from build123d import *

# Parameters (mm, degrees)
BOSS_EXTRUDE1_DEPTH = 11.1125
SKETCH3_W           = 6.35
SKETCH3_H           = 6.35
CUT_EXTRUDE1_DEPTH  = 6.35
SKETCH2_R           = 1.5875
CUT_EXTRUDE2_DEPTH  = 3.175
CUT_EXTRUDE3_REACH  = 19.451
SKETCH4_R           = 1.7859375


with BuildPart() as part:
    # Sketch1 → Boss-Extrude1 (new body)
    with BuildSketch(Plane.XY):
        Polygon((0, 0), (0, 7.62), (12.7, 7.62), (12.7, 4.445), (6.35, 4.445), (6.35, 0), align=None)
    extrude(amount=BOSS_EXTRUDE1_DEPTH)

    # Mirror1: part across plane


with BuildPart() as part_1:
    add(part.part)
    add(part.part.mirror(Plane(origin=(0, 0, 11.1125), x_dir=(0, 0, 1), z_dir=(-1, 0, 0))))

    # Sketch3 → Cut-Extrude1 (cut)
    with BuildSketch(Plane(origin=(0, 7.62, 0), x_dir=(1, 0, 0), z_dir=(0, 1, 0))):
        with Locations((0, -6.35)):
            Rectangle(SKETCH3_W, SKETCH3_H)
    extrude(amount=-CUT_EXTRUDE1_DEPTH, mode=Mode.SUBTRACT)

    # Sketch2 → Cut-Extrude2 (cut)
    with BuildSketch(Plane.ZY.offset(6.35)):
        with Locations(Location((5.55625, 2.8575, 0), (0, 0, 270))):
            Circle(SKETCH2_R)
    extrude(amount=-CUT_EXTRUDE2_DEPTH, mode=Mode.SUBTRACT)

    # Sketch4 → Cut-Extrude3 (cut, up to next)
    with BuildSketch(Plane.XZ.offset(-4.445), mode=Mode.PRIVATE) as cut_extrude3_sk1:
        with Locations((9.525, 2.8575)):
            Circle(SKETCH4_R)
    cut_extrude3_tool1 = extrude(cut_extrude3_sk1.sketch, amount=-CUT_EXTRUDE3_REACH, mode=Mode.PRIVATE) & part_1.part
    # Sketch4 → Cut-Extrude3 (cut, up to next)
    with BuildSketch(Plane.XZ.offset(-4.445), mode=Mode.PRIVATE) as cut_extrude3_sk2:
        with Locations((-9.525, 2.8575)):
            Circle(SKETCH4_R)
    cut_extrude3_tool2 = extrude(cut_extrude3_sk2.sketch, amount=-CUT_EXTRUDE3_REACH, mode=Mode.PRIVATE) & part_1.part
    add(cut_extrude3_tool1.solids().sort_by_distance((9.525, 4.445, 2.8575))[0], mode=Mode.SUBTRACT)
    add(cut_extrude3_tool2.solids().sort_by_distance((-9.525, 4.445, 2.8575))[0], mode=Mode.SUBTRACT)

    # Mirror2: part across plane


with BuildPart() as part_2:
    add(part_1.part)
    add(part_1.part.mirror(Plane(origin=(0, 0, 11.1125), x_dir=(1, 0, 0), z_dir=(0, 0, -1))))


solid = part_2.part
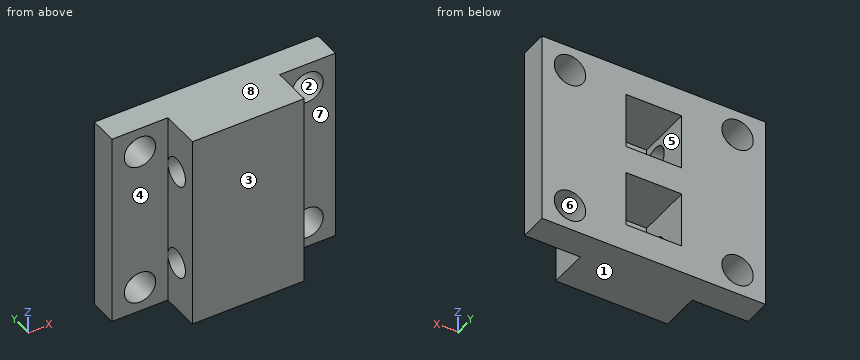
Model file for the job. Use its own axes, mm. Face numbers are marked on the shaded views. A direction names the side the tool comes from. Give positions to 0.01 mm unless a question says otherwise; leave off trailing zeros. Write each loop counter-clockwise with the first axis right and the second up, starting at its lowest first coordinate (ties: lowest second). Pieces come first, ordered by that corner, then holes. Notation, with made-up numbers: (14, -18.5) -> (27, -18.5) arc R11 cw to (27, -11.5) -> close; hole circle Ø9 at (-25, 49.25). An arc over 180 degrees is marked (long way). Write item = value, one per line.
(1) Slice it at C-C, the plane y = 5.5. Give the number of separate pieces and of enclosed holes in the cut face, then the cut area to 3 significant figures.
Determined:
separate_pieces = 1
enclosed_holes = 6
area = 444 mm2
(2) Slice it at D-D, the plane z = 20.25. Give the cut face in (x, y) (3 decimals).
Determined:
outline = (-12.7, 4.445) -> (-11.078, 4.445) -> (-11.078, 7.62) -> (-12.7, 7.62) -> close; (-7.972, 4.445) -> (-6.35, 4.445) -> (-6.35, 0) -> (6.35, 0) -> (6.35, 4.445) -> (7.972, 4.445) -> (7.972, 7.62) -> (-7.972, 7.62) -> close; (11.078, 4.445) -> (12.7, 4.445) -> (12.7, 7.62) -> (11.078, 7.62) -> close
(3) Mould opens along Z. For the marked faces 1, 2 and 3 say: released by +Z, released by -Z, zero draft, split by the parting line, or undercut.
Determined:
face_1 = released by -Z
face_2 = undercut
face_3 = zero draft
(4) Slice it at B-B, the plane x = -2. Give the cut face in (y, z) (3 decimals).
Determined:
outline = (0, 0) -> (7.62, 0) -> (7.62, 3.175) -> (1.27, 3.175) -> (1.27, 9.525) -> (7.62, 9.525) -> (7.62, 12.7) -> (1.27, 12.7) -> (1.27, 19.05) -> (7.62, 19.05) -> (7.62, 22.225) -> (0, 22.225) -> close
(5) Slice it at A-A, the plane z = 13.25. Give the cut face in (x, y) (3 decimals).
Determined:
outline = (-12.7, 4.445) -> (-6.35, 4.445) -> (-6.35, 0) -> (6.35, 0) -> (6.35, 4.445) -> (12.7, 4.445) -> (12.7, 7.62) -> (3.175, 7.62) -> (3.175, 1.27) -> (-3.175, 1.27) -> (-3.175, 7.62) -> (-12.7, 7.62) -> close
(6) Tool access for the marked faces 4, 5, 6, 7 and 8: list every direction of +Z, -Z, +X, -X, +Y, -Y with a clear straight run to the whole face (end or side of a thin tool).
Determined:
face_4 = +Z, -Z, -X, -Y
face_5 = +Y
face_6 = +Y, -Y
face_7 = +Z, -Z, +X, -Y
face_8 = +Z, +X, -X, +Y, -Y
(7) Probe line 1 along Z through (x, y) = (-3, 3) (3 decimals); line 2 along X through (y, z) = (6.25, 9.25) (3 decimals); line 3 along X through (y, z) = (6.25, 18.75) (3 decimals). List the from-to ranges inside material, lowest first.
Determined:
line_1 = 0 to 3.175, 9.525 to 12.7, 19.05 to 22.225
line_2 = -12.7 to -3.175, 3.175 to 12.7
line_3 = -12.7 to -11.201, -7.849 to -3.175, 3.175 to 7.849, 11.201 to 12.7
(8) Flat gauge pins, fed straight in: P1, Ø1.5, axis at y = 1, z = 12.5, coming from the -X side; P2, Ø4, axis at x = 9.52, z = 19.37, coming from the -Y side (3 decimals); P3, Ø3, axis at x = 9.52, z = 2.86, coming from the +Y side; P4, Ø1.9, axis at x = -0.5, z = 7.5, coming from the +Y side. Where does each tip first touch, or does it go through?
Determined:
P1 = -6.35
P2 = 4.445
P3 = through
P4 = 1.27
